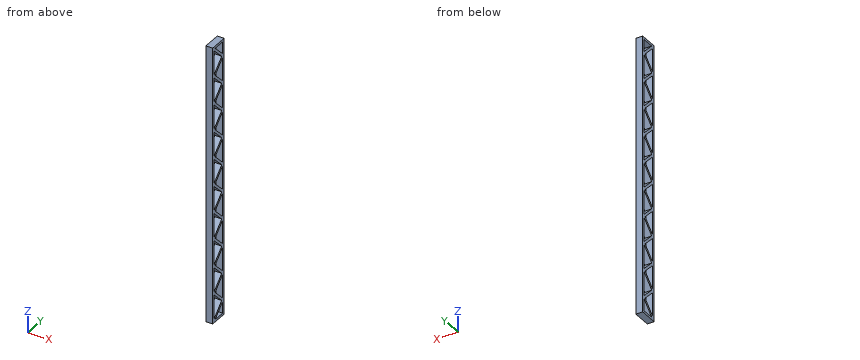
```python
from build123d import *

# Parameters (mm, degrees)
F1_DEPTH = 1.5


with BuildPart() as f1:
    # F0 (on Right) → F1 (new body)
    with BuildSketch(Plane.YZ):
        Polygon((4, 0), (0, 0), (0, -60), (0, -61), (0.353553, -61), (4, -61), (4, -60), align=None)
        Polygon((0.5, -54.853553), (3.146447, -57.5), (0.5, -60.146447), (0.5, -59.5), align=None, mode=Mode.SUBTRACT)
        Polygon((0.5, -48.853553), (3.146447, -51.5), (0.5, -54.146447), align=None, mode=Mode.SUBTRACT)
        Polygon((0.5, -42.853553), (3.146447, -45.5), (0.5, -48.146447), align=None, mode=Mode.SUBTRACT)
        Polygon((0.5, -36.853553), (3.146447, -39.5), (0.5, -42.146447), align=None, mode=Mode.SUBTRACT)
        Polygon((0.5, -30.853553), (3.146447, -33.5), (0.5, -36.146447), align=None, mode=Mode.SUBTRACT)
        Polygon((0.853553, -60.5), (3.5, -57.853553), (3.5, -59.5), (3.5, -60.5), align=None, mode=Mode.SUBTRACT)
        Polygon((3.5, -57.146447), (0.853553, -54.5), (3.5, -51.853553), align=None, mode=Mode.SUBTRACT)
        Polygon((3.5, -51.146447), (0.853553, -48.5), (3.5, -45.853553), align=None, mode=Mode.SUBTRACT)
        Polygon((3.5, -45.146447), (0.853553, -42.5), (3.5, -39.853553), align=None, mode=Mode.SUBTRACT)
        Polygon((3.5, -39.146447), (0.853553, -36.5), (3.5, -33.853553), align=None, mode=Mode.SUBTRACT)
        Polygon((3.5, -33.146447), (0.853553, -30.5), (3.5, -27.853553), align=None, mode=Mode.SUBTRACT)
        Polygon((0.5, -24.853553), (3.146447, -27.5), (0.5, -30.146447), align=None, mode=Mode.SUBTRACT)
        Polygon((0.5, -18.853553), (3.146447, -21.5), (0.5, -24.146447), align=None, mode=Mode.SUBTRACT)
        Polygon((0.5, -12.853553), (3.146447, -15.5), (0.5, -18.146447), align=None, mode=Mode.SUBTRACT)
        Polygon((0.5, -6.853553), (3.146447, -9.5), (0.5, -12.146447), align=None, mode=Mode.SUBTRACT)
        Polygon((0.5, -6.146447), (0.5, -0.853553), (3.146447, -3.5), align=None, mode=Mode.SUBTRACT)
        Polygon((3.5, -27.146447), (0.853553, -24.5), (3.5, -21.853553), align=None, mode=Mode.SUBTRACT)
        Polygon((3.5, -21.146447), (0.853553, -18.5), (3.5, -15.853553), align=None, mode=Mode.SUBTRACT)
        Polygon((3.5, -15.146447), (0.853553, -12.5), (3.5, -9.853553), align=None, mode=Mode.SUBTRACT)
        Polygon((0.853553, -6.5), (3.5, -3.853553), (3.5, -9.146447), align=None, mode=Mode.SUBTRACT)
        Polygon((0.853553, -0.5), (3.5, -0.5), (3.5, -3.146447), align=None, mode=Mode.SUBTRACT)
    extrude(amount=F1_DEPTH)


solid = f1.part
```
Work out the finished part from the listing and answer in its coordinate system (mm). Round coordinates to 2 decimals unless told otherwise and drop trailing zeros. Write each loop counter-clockwise with the first axis right and the second up, starting at its lowest first coordinate (ties: lowest second). Pieces come first, ordered by that corner, then holes.
1) A cutting plane is placed at A-A on z = -56. Determine the outline of the cut face in (x, y), and give its area (3 significant figures).
2) A cutting plane is placed at B-B on x = 0.8. Give the number of separate pieces and of enclosed holes in the cut face, and give its area (3 significant figures).
3) Consider probe 1 along Y at (x, z) = (1.35, -59); probe 2 along Y at (x, z) = (0.3, -14.5). Determine where each line is inside the solid, lowest interval first.
Entries:
1. outline: (0, 0) - (1.5, 0) - (1.5, 0.5) - (0, 0.5) - close; (0, 1.65) - (1.5, 1.65) - (1.5, 2.35) - (0, 2.35) - close; (0, 3.5) - (1.5, 3.5) - (1.5, 4) - (0, 4) - close
1. area: 2.56 mm2
2. separate pieces: 1
2. enclosed holes: 21
2. area: 104 mm2
3. probe 1: y = 0 to 0.5, 1.65 to 2.35, 3.5 to 4
3. probe 2: y = 0 to 0.5, 2.15 to 2.85, 3.5 to 4
